from build123d import *

# Parameters (mm, degrees)
SZKIC1_R                    = 12
DODANIE_WYCI_GNI_CIE1_DEPTH = 15
SZKIC2_R                    = 20
WYTNIJ_WYCI_GNI_CIE1_DEPTH  = 7.5
ZAOKR_GLENIE1_R             = 10


with BuildPart() as part:
    # Szkic1 → Dodanie-wyciągnięcie1 (new body)
    with BuildSketch(Plane.XY):
        with BuildLine():
            Line((0, -20), (0, -490))
            ThreePointArc((0, -490), (-281.052453812, -401.384501702), (-460.449384185, -167.58987023))
            Line((-460.449384185, -167.58987023), (-18.793852416, -6.840402867))
            ThreePointArc((-18.793852416, -6.840402867), (11.471528727, 16.383040886), (0, -20))
        make_face()
        Circle(SZKIC1_R, mode=Mode.SUBTRACT)
    extrude(amount=DODANIE_WYCI_GNI_CIE1_DEPTH)

    # Szkic2 → Wytnij-wyciągnięcie1 (cut)
    with BuildSketch(Plane(origin=(0, 0, 0), x_dir=(-1, 0, 0), z_dir=(0, 0, -1))):
        Circle(SZKIC2_R)
    extrude(amount=-WYTNIJ_WYCI_GNI_CIE1_DEPTH, mode=Mode.SUBTRACT)

    # Zaokrąglenie1
    zaokr_glenie1_edges = [part.edges().sort_by_distance(p)[0] for p in [
        (-18.793852416, -6.840402867, 11.25),
    ]]
    fillet(zaokr_glenie1_edges, radius=ZAOKR_GLENIE1_R)


solid = part.part
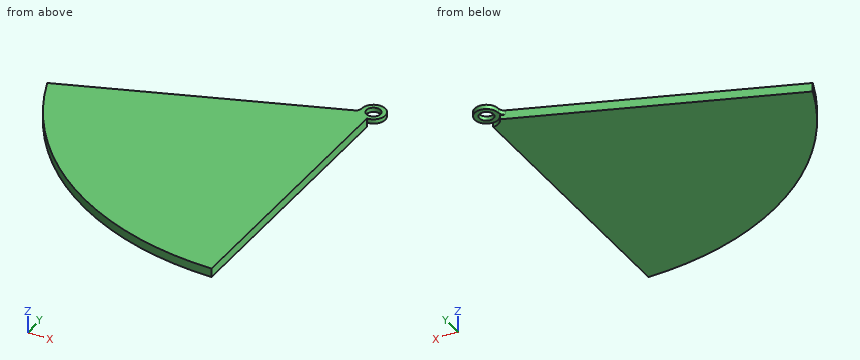
Geometry: final body of the model. Coordinates: model frame, mm. Give positions to 0.01 mm unless a question says otherwise; leave off trailing zeros. Write each loop counter-clockwise with the first axis right and the second up, starting at its lowest first coordinate (ties: lowest second). Pieces come first, ordered by that corner, then holes. Notation, with made-up numbers: (62.5, 53) -> (75.5, 53) arc R13 cw to (75.5, 57) -> close; hole circle Ø9 at (-35, 16.5). An arc over 180 degrees is marked (long way). Answer in a Markdown table with one row per item.
(1) Ray query, line 1 along X through (y, z) = (0, 10); line 2 along Y through (x, z) = (-286, 1.5); line 3 along X through (y, z) = (-414, 4). Return the intervals inside material, ascending. Write a range as [from, to].
Answers below:
| item | result |
|---|---|
| line 1 | [-20, -12], [12, 20] |
| line 2 | [-397.87, -104.1] |
| line 3 | [-262.11, 0] |
(2) Section query A-A on z = 10.25. Return loops of the section in (x, y), then the cut area to 3 significant figures.
Answers below:
| item | result |
|---|---|
| outline | (-460.45, -167.59) arc R490 ccw to (0, -490) -> (0, -20) arc R20 ccw (long way) to (-20, -0.18) arc R10 cw to (-26.58, -9.67) -> close; hole circle Ø24 at (0, 0) |
| area | 147,000 mm^2 |
(3) Pin query (flat end, axial travel): pin 1 (2 mm diameter, centred on x = -277.5, z = 12.5, fed in from +Y); pin 2 (7.5 mm diameter, centred on y = -338, z = 6, fed in from +X); pin 3 (3 mm diameter, centred on y = -297.5, z = 11.5, fed in from -X). Return the tip coordinate at first contact, or that it passes through.
Answers below:
| item | result |
|---|---|
| pin 1 | y = -100.64 |
| pin 2 | x = 0 |
| pin 3 | x = -390.49 |
(4) Section query B-B on x = -404. Return loops of the section in (y, z).
Answers below:
| item | result |
|---|---|
| outline | (-277.28, 0) -> (-147.04, 0) -> (-147.04, 15) -> (-277.28, 15) -> close |
(5) Section query C-C on y = -91. Return loops of the section in (x, z), then the cut area to 3 significant figures.
Answers below:
| item | result |
|---|---|
| outline | (-250.02, 0) -> (0, 0) -> (0, 15) -> (-250.02, 15) -> close |
| area | 3,750 mm^2 |
